The model under review builds one solid part; all positions refer to its coordinate system, in mm. A direction names the side the tool comes from. Coordinates: 2 decimals unless noted, no trailing zeros. Loops run counter-clockwise (first coordinate to the right, second up) from the corner with the lowest first, then second, coordinate; pieces in that order, holes last. Notation, with made-up numbers: M 57,-30 L 74,-30 A25 cw 74,-11 Z; hole C -16,-23 d1. An arc over 180 degrees is marked long. One line per item, written item: value.
```python
from build123d import *

# Parameters (mm, degrees)
F0_W     = 160
F0_H     = 160
F0_W_2   = 130
F0_H_2   = 140
F1_DEPTH = 40
F2_W     = 160
F2_H     = 160
F3_DEPTH = 15


with BuildPart() as f1:
    # F0 (on Top) → F1 (new body)
    with BuildSketch(Plane.XY):
        Rectangle(F0_W, F0_H)
        Rectangle(F0_W_2, F0_H_2, mode=Mode.SUBTRACT)
    extrude(amount=F1_DEPTH)

    # F2 (on Top) → F3 (join)
    with BuildSketch(Plane.XY):
        Rectangle(F2_W, F2_H)
    extrude(amount=-F3_DEPTH)


solid = f1.part
```
(1) Draft analysis for pull direction X (two halves, no side actions). For faces 1 (the face through (-1, -70, 20)), 2 (the face through (-1, 70, 20)), 3 (the face through (-80, -1, 13)), 4 (the face through (-66, 0, 40)), state which applies: pulls with the +X half, pulls with the -X half, needs draft (parallel to the pull), parting line crosses it, or undercut.
Checks:
face 1: undercut
face 2: undercut
face 3: pulls with the -X half
face 4: needs draft
(2) Add section A-A on z = 28. State the section outline as (x, y) points.
Checks:
outline: M -80,-80 L 80,-80 L 80,80 L -80,80 Z; hole M -65,-70 L 65,-70 L 65,70 L -65,70 Z
(3) Add section C-C on x = 39. State the section outline as (y, z) points, then the cut area to 3 significant figures.
Checks:
outline: M -80,-15 L 80,-15 L 80,40 L 70,40 L 70,0 L -70,0 L -70,40 L -80,40 Z
area: 3,200 mm^2
(4) To check wall thickness, follow L1, parallel to X at y = -14.5, z = 16; L2, parallel to Y at x = -37, z = 28.5; L3, parallel to Z at x = -16.5, y = 24.5. State the ranges of each line that lie inside material, in increasing order. Write a range as [from, to].
Checks:
L1: [-80, -65], [65, 80]
L2: [-80, -70], [70, 80]
L3: [-15, 0]
(5) Insertion check: pin 1 Ø6 at (x, y) = (-51, -53.5) entering from +Z. The pin has a flat end and moves straight along its axis. Give the tip position at first contact, or say it passes through.
Checks:
pin 1: z = 0
(6) Add section B-B on y = 5.5. State the section outline as (x, z) points.
Checks:
outline: M -80,-15 L 80,-15 L 80,40 L 65,40 L 65,0 L -65,0 L -65,40 L -80,40 Z
(7) Tool access review of faces 5 (the face through (-1, 80, 13)), 6 (the face through (-1, 1, 0)): name each direction out of +Z, -Z, +X, -X, +Y, -Y from which nothing blocks a thin tool from reaching the whole face with its end or side.
Checks:
face 5: +Z, -Z, +X, -X, +Y
face 6: +Z
